Here's the drawing with two shaded views (mm, measured from the low corner). I have some questions. A direction names the side the tool comes from. Round coordinates to 2 decimals unless told otherwise and drop trailing zeros. Loops run counter-clockwise (first coordinate to the right, second up) from the corner with the lowest first, then second, coordinate; pieces in that order, holes last. Notation, with made-up numbers: M 7.25,80.5 L 25.25,80.5 A26 ccw 25.25,112.5 Z; hole C -29.5,88.5 d7. An arc over 180 degrees is marked long. Answer as a JSON object with one key per item and string values.
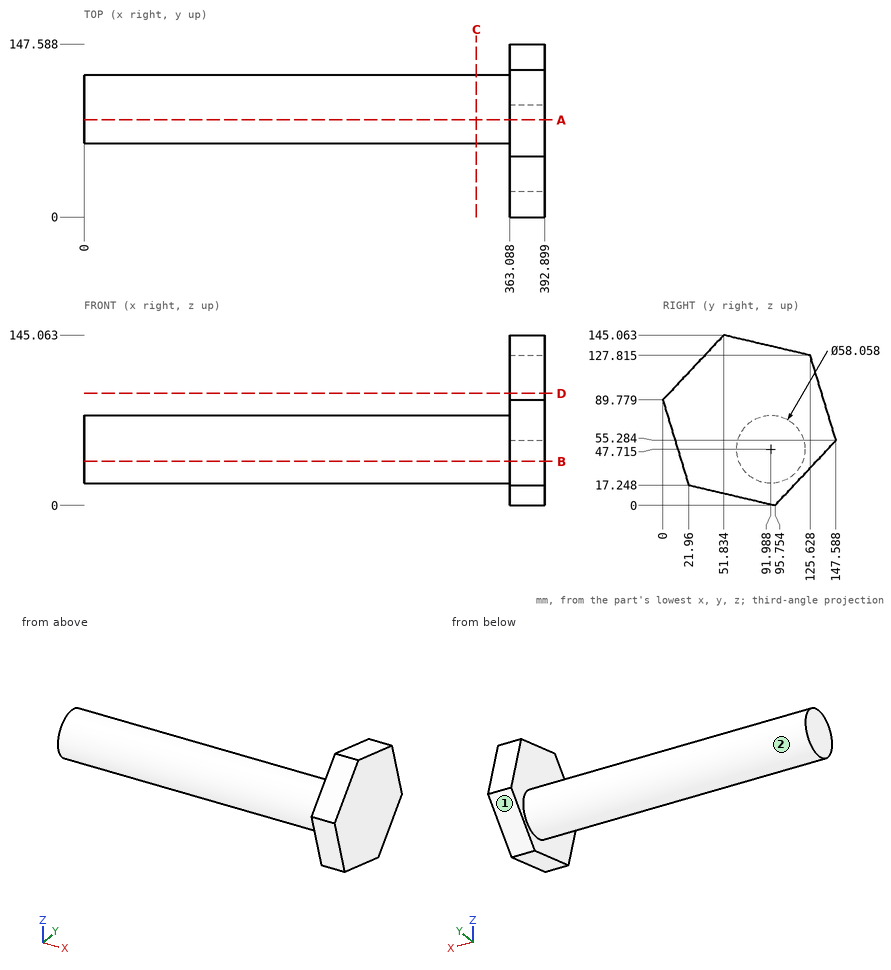
Item 1: For P1, Ø10, axis at x = 200, y = 67.5, coming from the +Z side; P2, Ø10, axis at y = 130.5, z = 52, coming from the -X side; P3, Ø4, axis at x = 205.5, y = 82, coming from the -Z side, each with a flat end and sliding along its axis, tell me the tip position at first contact or that it passes through.
Solution:
{"P1": "stops at z = 69.23", "P2": "stops at x = 363.09", "P3": "stops at z = 19.81"}
Item 2: I want a section at B-B on z = 37.5. List the corners of the cut face in (x, y) for me (1 decimal), plus the area to 3 significant figures.
Solution:
{"outline": "M 0,64.8 L 363.1,64.8 L 363.1,15.8 L 392.9,15.8 L 392.9,130.9 L 363.1,130.9 L 363.1,119.2 L 0,119.2 Z", "area": "23,200 mm2"}
Item 3: I want a section at C-C on x = 334.5. List the corners of the cut face in (y, z) for me (1 decimal), plus the area to 3 significant figures.
Solution:
{"outline": "C 92,47.7 d58.1", "area": "2,650 mm2"}
Item 4: I want a section at D-D on z = 95.5. List the corners of the cut face in (x, y) for me.
Solution:
{"outline": "M 363.09,5.36 L 392.9,5.36 L 392.9,135.41 L 363.09,135.41 Z"}
Item 5: If I drill on L1, parallel to X at y = 88.5, z = 127; L2, parallel to Z at x = 174, y = 95; L3, parallel to Y at x = 263.5, z = 38, over which ranges is the centre line in solid material (lowest first)? Write a range as from..to.
Solution:
{"L1": "x = 363.09..392.9", "L2": "z = 18.84..76.59", "L3": "y = 64.63..119.34"}
Item 6: For the marked faces 1 and 2, which set-ups out of +Z, -Z, +X, -X, +Y, -Y let a thin tool reach every point of the face, with its end or its side?
Solution:
{"face 1": "-Z, +X, -X, +Y", "face 2": "-X"}
Item 7: I want a section at A-A on y = 83. List the corners of the cut face in (x, z) for me.
Solution:
{"outline": "M 0,20.11 L 363.09,20.11 L 363.09,2.98 L 392.9,2.98 L 392.9,137.78 L 363.09,137.78 L 363.09,75.32 L 0,75.32 Z"}
